Read the model definition and answer for the solid it produces. Units are mm, in the model's axes. A direction names the side the tool comes from. Coordinates: 2 decimals unless noted, no trailing zeros. Write each loop counter-clockwise with the first axis right and the second up, starting at its lowest first coordinate (ties: lowest second). Pieces come first, ordered by that corner, then holes. Notation, with made-up numbers: (12, 4.5) -> (33, 4.5) arc R31 ccw to (33, 31.5) -> close; hole circle Ø3 at (-4, -35.5). An arc over 180 degrees is marked (long way). Answer as a JSON object with one key per item and string values. Group by question number.
(1) Flat-ended cylindrical pins translate along their axes: P1, Ø5, axis at x = 10, y = 7.5, coming from the +Z side; P2, Ø2, axis at y = 13, z = 3.5, coming from the -X side; P3, Ø2, axis at y = 13, z = 2.5, coming from the +X side. Find the tip coordinate at first contact, or state that the pin passes through.
(2) Find section A-A (x = 10). Give the vertices of the cut face in (y, z).
(3) Find section D-D (x = 62.5). Give the vertices of the cut face in (y, z).
(4) Straight lines are drawn through the part: L1, parallel to X at y = 7.5, z = 11.25; L2, parallel to X at y = 7.5, z = 7.5; L3, parallel to X at y = 5.25, z = 7.75. For each, find the intervals that lie inside material, in ascending order.
(5) Which of the six approach directions +Z, -Z, +X, -X, +Y, -Y give full straight-line access (tool end or side, diameter ignored) to faces 4 (the face through (1.141, 1.203, 7.605)), 5 (the face through (3.242, 7.591, 5.435))?
(6) Find section B-B (z = 3.5). Give the vertices of the cut face in (x, y).
(7) For a pull along Y with two mould halves and no side action, classify faces 1 (the face through (68.797, 1.141, 7.605)), 2 (the face through (13.966, 8.021, 7.605)), 3 (the face through (70, 7, 7)) as +Y half, -Y half, draft (parallel to the pull), parting line (faces both ways), or undercut.
(8) Find section C-C (y = 6.25). Give the vertices of the cut face in (x, z), then the cut area to 3 significant figures.
Solid Edge part; units mm, degrees
sketch "Sketch1" plane through (0, 0, 0) normal (0, 0, 1) x (1, 0, 0)
  line L0 (70, 0) -> (70, 15)
  line L1 (70, 15) -> (0, 15)
  line L2 (0, 15) -> (0, 0)
  line L3 (0, 0) -> (70, 0)
extrude "Protrusion1" add sketch "Sketch1" along normal blind 15
hole "Bohrung_1" at (10, 7.5, 15) direction (0, 0, -1) diameter 8 end through all
hole "Bohrung_2" at (62.5, 7.5, 15) direction (0, 0, -1) diameter 4.917 end through all
hole "Bohrung_3" at (0, 7.5, 7.5) direction (1, 0, 0) diameter 4.134 end up to next
fillet "Verrundung_1" radius 4 4 edges at (70, 15, 7.5) (70, 0, 7.5) (0, 15, 7.5) (0, 0, 7.5)
Results below:
{
 "1": {"P1": "passes through", "P2": "stops at x = 0.13", "P3": "stops at x = 69.87"},
 "2": {"outline": "(0, 0) -> (3.5, 0) -> (3.5, 15) -> (0, 15) -> close; (11.5, 0) -> (15, 0) -> (15, 15) -> (11.5, 15) -> close"},
 "3": {"outline": "(0, 0) -> (5.04, 0) -> (5.04, 15) -> (0, 15) -> close; (9.96, 0) -> (15, 0) -> (15, 15) -> (9.96, 15) -> close"},
 "4": {"L1": "x = 0 to 6, 14 to 60.04, 64.96 to 70", "L2": "x = 14 to 60.04, 64.96 to 70", "L3": "x = 0 to 6.69, 13.31 to 61.51, 63.49 to 70"},
 "5": {"face 4": "+Z, -Z, -X, -Y", "face 5": "-X"},
 "6": {"outline": "(0, 4) arc R4 ccw to (4, 0) -> (66, 0) arc R4 ccw to (70, 4) -> (70, 11) arc R4 ccw to (66, 15) -> (4, 15) arc R4 ccw to (0, 11) -> close; hole circle Ø8 at (10, 7.5); hole circle Ø4.92 at (62.5, 7.5)"},
 "7": {"face 1": "-Y half", "face 2": "undercut", "face 3": "draft"},
 "8": {"outline": "(0, 0) -> (6.2, 0) -> (6.2, 5.85) -> (0, 5.85) -> close; (0, 9.15) -> (6.2, 9.15) -> (6.2, 15) -> (0, 15) -> close; (13.8, 0) -> (60.38, 0) -> (60.38, 15) -> (13.8, 15) -> close; (64.62, 0) -> (70, 0) -> (70, 15) -> (64.62, 15) -> close", "area": "852 mm2"}
}
